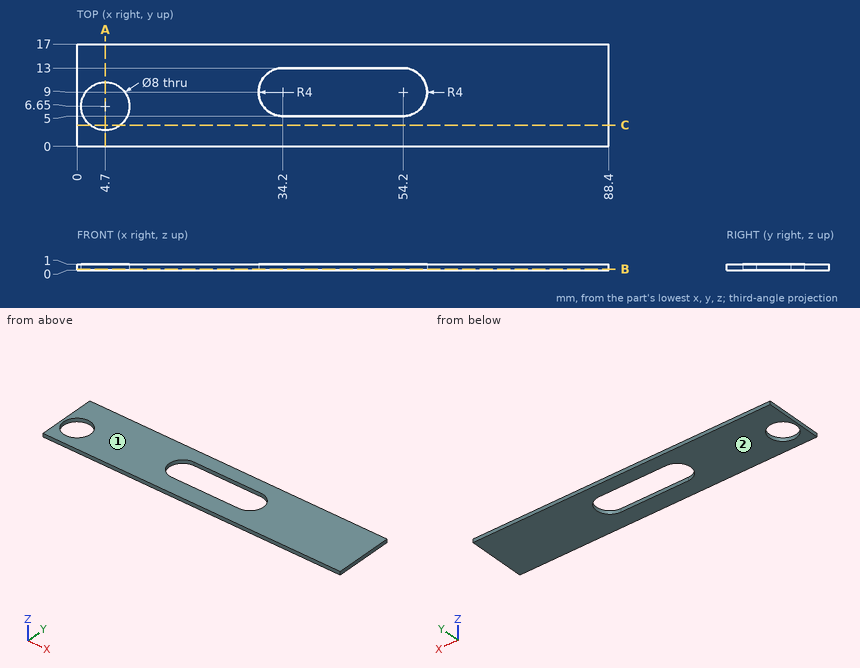
Check sheet for the drawn part. Datum: minimum x, y, z corner. Units: mm. Give positions to 0.01 mm unless a question says otherwise; leave off trailing zeros. Order: outer loops, then holes, each group sorted by start corner. A loop starts at its lowest first (then second) coordinate and runs counter-clockwise, first axis right, second up.
1. Draft check along Z on the marked faces 1 and 2. Enter one of: pulls with the +Z half, pulls with the -Z half, needs draft (parallel to the pull), parting line crosses it, or undercut.
Completed:
face 1: pulls with the +Z half
face 2: pulls with the -Z half
2. Sectioned sample at C-C (y = 3.5). Record the boundary of the cut face in (x, z).
Completed:
outline: (0, 0) - (2.23, 0) - (2.23, 1) - (0, 1) - close; (7.17, 0) - (88.4, 0) - (88.4, 1) - (7.17, 1) - close
3. Sectioned sample at A-A (x = 4.7). Record the boundary of the cut face in (y, z).
Completed:
outline: (0, 0) - (2.65, 0) - (2.65, 1) - (0, 1) - close; (10.65, 0) - (17, 0) - (17, 1) - (10.65, 1) - close
4. Sectioned sample at B-B (z = 0.2). Record the boundary of the cut face in (x, y).
Completed:
outline: (0, 0) - (88.4, 0) - (88.4, 17) - (0, 17) - close; hole circle Ø8 at (4.7, 6.65); hole (34.2, 5) - (54.2, 5) arc R4 ccw to (54.2, 13) - (34.2, 13) arc R4 ccw to start
5. Scan lines: line 1 (Y direction, x = 38.5, z = 0.9); line 2 (Y direction, x = 4.7, z = 0.7); line 3 (X direction, y = 12.5, z = 0.55). Record each from-to range of solid material in increasing order.
Completed:
line 1: y = 0 to 5, 13 to 17
line 2: y = 0 to 2.65, 10.65 to 17
line 3: x = 0 to 32.26, 56.14 to 88.4
